Autodesk Inventor part; units mm, degrees
ref_plane "YZ Plane" through (0, 0, 0) normal (1, 0, 0) x (0, 1, 0)
ref_plane "XZ Plane" through (0, 0, 0) normal (0, 1, 0) x (-1, 0, 0)
ref_plane "XY Plane" through (0, 0, 0) normal (0, 0, 1) x (1, 0, 0)
sketch "Sketch1" plane through (0, 0, 0) normal (0, 0, 1) x (1, 0, 0)
  circle A0 centre (0, 0) radius 4.1
  arc A1 (-7.5, 0) -> (7.5, 0) centre (0, 0) ccw
  circle A2 centre (0, 55) radius 4.1
  arc A3 (7.5, 55) -> (-7.5, 55) centre (0, 55) ccw
  line L0 (-7.5, 55) -> (-7.5, 0)
  circle A4 centre (7.5, 45) radius 5
  line L1 (7.5, 0) -> (7.5, 40)
  line L2 (7.5, 50) -> (7.5, 55)
  dimension "d0" = 55
  dimension "d1" = 15
  dimension "d2" = 8.2
  dimension "d3" = 8.2
  dimension "d4" = 10
  dimension "d5" = 10
  dimension "d8" = 15
  dimension "d10" = 15
extrude "Extrusion1" add sketch "Sketch1" along normal blind 3 contours A0 | L0 A3 L2 A4 L1 A1
fillet "Fillet1" radius 2 2 edges at (7.5, 50, 1.5) (7.5, 40, 1.5)
equation "\"d3\" = d2"
equation "\"d5\" = d4"
equation "\"d8\" = d10"
properties part number "Jambe" material "Aluminum 6061"
Could you check a few things on this model? Use its own coordinates, in mm. A direction names the side the tool comes from. Round coordinates to 2 decimals unless told otherwise and drop trailing zeros. Loops run counter-clockwise (first coordinate to the right, second up) from the corner with the lowest first, then second, coordinate; pieces in that order, holes last. Notation, with made-up numbers: (-18.5, -5.75) -> (21.5, -5.75) arc R22 cw to (21.5, 9.25) -> close; hole circle Ø4 at (58, 57.25). An arc over 180 degrees is marked (long way). Put each result on its own line as item: value.
Q1. I want a section at D-D on x = -5.75. Write out the boundary of the cut face in (y, z), and give its area (3 significant figures).
Checks:
outline: (-4.82, 0) -> (59.82, 0) -> (59.82, 3) -> (-4.82, 3) -> close
area: 194 mm2
Q2. Thinking about a two-plate mould opening in Y: for faces 1 (the cylindrical face through (-0.534, 50.935, 1.479)), 2 (the flat face through (7.5, 53, 1)), 3 (the cylindrical face through (-0.16, 62.5, 1.48)), which applies, pulls with the +Y half, pulls with the -Y half, needs draft (parallel to the pull), parting line crosses it, or undercut?
Checks:
face 1: undercut
face 2: needs draft
face 3: pulls with the +Y half
Q3. I want a section at A-A on x = 0. Write out the boundary of the cut face in (y, z).
Checks:
outline: (-7.5, 0) -> (50.9, 0) -> (50.9, 3) -> (-7.5, 3) -> close; (59.1, 0) -> (62.5, 0) -> (62.5, 3) -> (59.1, 3) -> close
Q4. I want a section at B-B on z = 0.5. Write out the boundary of the cut face in (x, y), and give its area (3 significant figures).
Checks:
outline: (-7.5, 0) arc R7.5 ccw to (7.5, 0) -> (7.5, 38.29) arc R2 ccw to (6.07, 40.21) arc R5 cw to (6.07, 49.79) arc R2 ccw to (7.5, 51.71) -> (7.5, 55) arc R7.5 ccw to (-7.5, 55) -> close; hole circle Ø8.2 at (0, 55)
area: 909 mm2
Q5. I want a section at C-C on x = -3. Write out the boundary of the cut face in (y, z), and give its area (3 significant figures).
Checks:
outline: (-6.87, 0) -> (52.21, 0) -> (52.21, 3) -> (-6.87, 3) -> close; (57.79, 0) -> (61.87, 0) -> (61.87, 3) -> (57.79, 3) -> close
area: 189 mm2
Q6. Which directions (+Z, -Z, +X, -X, +Y, -Y) give clear straight access to the entire face, cutting with the end or side of a thin tool? Please do faces 4 (the cylindrical face through (7.093, 50.499, 1.521)), 5 (the flat face through (-7.5, 28, 1)).
Checks:
face 4: +Z, -Z, +X
face 5: +Z, -Z, -X, +Y, -Y
Q7. Please list where these lines run through material, in increasing order: line 1 (Y direction, x = 0, z = 1.8); line 2 (Y direction, x = -1.5, z = 1.2); line 3 (Y direction, x = -4.75, z = 2.2). Write a range as from..to.
Checks:
line 1: -7.5..50.9, 59.1..62.5
line 2: -7.35..51.18, 58.82..62.35
line 3: -5.8..60.8
